```python
from build123d import *

# Parameters (mm, degrees)
F0_W      = 762
F0_H      = 609.6
F1_DEPTH  = 914.4
F2_R      = 101.6
F2_R_2    = 76.2
F3_DEPTH  = 7.62
F2_W      = 762
F2_H      = 88.9
F4_DEPTH  = 279.4
F5_W      = 762
F5_H      = 47.1075362206
F5_H_2    = 643.9726948738
F5_H_3    = 166.3404107094
F6_DEPTH  = 30.48
F8_DEPTH  = 63.5
F9_R      = 25.4
F10_W     = 762
F10_H     = 160.2732217789
F11_DEPTH = 25.4
F12_R     = 31.75
F13_DEPTH = 30.48
F12_W     = 194.5324838161
F12_H     = 87.0171510696
F14_DEPTH = 6.35
F15_W     = 533.4
F15_H     = 386.08
F16_DEPTH = 762.762


with BuildPart() as f1:
    # F0 (on Top) → F1 (new body)
    with BuildSketch(Plane.XY):
        Rectangle(F0_W, F0_H)
    extrude(amount=F1_DEPTH)

    # F2 (on face) → F3 (join)
    with BuildSketch(Plane.XY.offset(914.4)):
        with Locations((-191.7613367384, 87.7341254172)):
            Circle(F2_R)
        with Locations((-191.7613367384, -176.6341254172)):
            Circle(F2_R_2)
        with Locations((191.7613367384, 87.7341254172)):
            Circle(F2_R_2)
        with Locations((191.7613367384, -176.6341254172)):
            Circle(F2_R)
    extrude(amount=F3_DEPTH)

    # F2 (on face) → F4 (join)
    with BuildSketch(Plane.XY.offset(914.4)):
        with Locations((0, 260.35)):
            Rectangle(F2_W, F2_H)
    extrude(amount=F4_DEPTH)

    # F5 (on face) → F6 (join)
    with BuildSketch(Plane.XZ.offset(304.8)):
        with Locations((0, 890.8462318897)):
            Rectangle(F5_W, F5_H)
        with Locations((0, 523.5575735569)):
            Rectangle(F5_W, F5_H_2)
        with Locations((0, 83.1702053547)):
            Rectangle(F5_W, F5_H_3)
    extrude(amount=F6_DEPTH)

    # F7 (on face) → F8 (join)
    with BuildSketch(Plane.XY.offset(845.5439209938)):
        with BuildLine():
            Line((-210.1894695859, -335.28), (-327.3042738438, -335.28))
            ThreePointArc((-327.3042738438, -335.28), (8.59336555, -451.5700550038), (344.4910049438, -335.28))
            Line((344.4910049438, -335.28), (227.376200686, -335.28))
            ThreePointArc((227.376200686, -335.28), (8.5933655501, -388.0700550038), (-210.1894695859, -335.28))
        make_face()
    extrude(amount=-F8_DEPTH)

    # F9
    f9_edges = [f1.edges().sort_by_distance(p)[0] for p in [
        (8.593366, -451.570055, 845.543921),
        (8.593366, -451.570055, 782.043921),
    ]]
    fillet(f9_edges, radius=F9_R)

    # F10 (on face) → F11 (join)
    with BuildSketch(Plane.XZ.offset(-215.9)):
        with Locations((0, 1113.6633891106)):
            Rectangle(F10_W, F10_H)
    extrude(amount=F11_DEPTH)

    # F12 (on face) → F13 (join)
    with BuildSketch(Plane.XZ.offset(-190.5)):
        with Locations((-304.8, 1113.6633891106)):
            Circle(F12_R)
        with Locations((-190.5, 1113.6633891106)):
            Circle(F12_R)
        with Locations((190.5, 1113.6633891106)):
            Circle(F12_R)
        with Locations((304.8, 1113.6633891106)):
            Circle(F12_R)
    extrude(amount=F13_DEPTH)

    # F12 (on face) → F14 (cut)
    with BuildSketch(Plane.XZ.offset(-190.5)):
        with Locations((0, 1113.6633891106)):
            Rectangle(F12_W, F12_H)
    extrude(amount=-F14_DEPTH, mode=Mode.SUBTRACT)

    # F15 (on face) → F16 (cut)
    with BuildSketch(Plane(origin=(0, 0, 0), x_dir=(1, 0, 0), z_dir=(0, 0, -1))):
        with Locations((12.7, 15.24)):
            Rectangle(F15_W, F15_H)
    extrude(amount=-F16_DEPTH, mode=Mode.SUBTRACT)


solid = f1.part
```
The listing builds one solid part. Answer for the finished solid, in the listing's coordinates (mm). A direction names the side the tool comes from. Round coordinates to 2 decimals unless told otherwise and drop trailing zeros. Write each loop counter-clockwise with the first axis right and the second up, starting at its lowest first coordinate (ties: lowest second). Pieces come first, ordered by that corner, then holes. Notation, with made-up numbers: (49.25, -10) -> (75.25, -10) arc R13 cw to (75.25, 5) -> close; hole circle Ø4 at (26.25, -19). An arc over 180 degrees is marked (long way). Use CSV: the item, a comma, the result in double quotes. Start each with the question number.
(1) Consider L1, parallel to Z at x = -193, y = -333; L2, parallel to Y at x = 129.5, z = 529.5; L3, parallel to X at y = -15.5, z = 757.5. Determine where each line is inside the solid, lowest interval first. Write a range as from..to.
(2) Each of these flat-tipped pins is pushed along its axis until it touches: pin 1 (5 mm diameter, centred on x = 291, y = 84.5, fed in from +Z); pin 2 (2 mm diameter, centred on x = 158.5, z = 227.5, fed in from -Y); pin 3 (19 mm diameter, centred on x = -297.5, z = 1103.5, fed in from -Y). Where does it stop, or does it pass through?
(3) Section B-B on y = -124 is taken. Give the vertices of the cut face in (x, z), then the cut area to 3 significant figures.
(4) Section C-C on z = 959.5 is taken. Give the vertices of the cut face in (x, y).
(5) Which of the six approach directions +Z, -Z, +X, -X, +Y, -Y give full straight-line access (tool end or side, diameter ignored) to faces 4 (the face through (-5, 203, 1033.527)), 5 (the face through (-173.431, 175.473, 1140.435)), 6 (the face through (-305, 160.02, 1114)), 7 (the face through (4, -390, 782.044))?
(6) The mould has two halves that part along Y. Classify faces 1 (the face through (191, 89, 922.02)), 2 (the face through (9, 177.8, 376)), 3 (the face through (3.524, -451.546, 813.883)): released by +Y, released by -Y, zero draft, split by the parting line, or undercut.
(7) Section A-A on z = 430.5 is taken. Give the vertices of the cut face in (x, y).
A:
1,L1,"z = 0..166.34, 201.57..845.54, 867.29..914.4"
1,L2,"y = -335.28..-208.28, 177.8..304.8"
1,L3,"x = -381..-254, 279.4..381"
2,pin 1,"stops at z = 914.4"
2,pin 2,"stops at y = -335.28"
2,pin 3,"stops at y = 160.02"
3,outline,"(-381, 0) -> (-254, 0) -> (-254, 762.76) -> (279.4, 762.76) -> (279.4, 0) -> (381, 0) -> (381, 914.4) -> (278.66, 914.4) -> (278.66, 922.02) -> (104.86, 922.02) -> (104.86, 914.4) -> (-136.66, 914.4) -> (-136.66, 922.02) -> (-246.86, 922.02) -> (-246.86, 914.4) -> (-381, 914.4) -> close"
3,area,"292,000 mm²"
4,outline,"(-381, 215.9) -> (381, 215.9) -> (381, 304.8) -> (-381, 304.8) -> close"
5,face 4,"+X, -X, -Y"
5,face 5,"-Y"
5,face 6,"+Z, +X, -X, -Y"
5,face 7,"-Z, +X, -X, -Y"
6,face 1,"zero draft"
6,face 2,"undercut"
6,face 3,"released by -Y"
7,outline,"(-381, -335.28) -> (381, -335.28) -> (381, 304.8) -> (-381, 304.8) -> close; hole (-254, -208.28) -> (279.4, -208.28) -> (279.4, 177.8) -> (-254, 177.8) -> close"
